The listing builds one solid part. Answer for the finished solid, in the listing's coordinates (mm). Face numbers are marked on the shaded views. A direction names the side the tool comes from. Round coordinates to 2 decimals unless told otherwise and drop trailing zeros. Loops run counter-clockwise (first coordinate to the right, second up) from the corner with the lowest first, then second, coordinate; pieces in that order, holes last. Notation, with made-up numbers: (58, -22) - (84, -22) arc R29 cw to (84, 14) - close; hole circle Ø1 at (-38, 7.25). An arc over 180 degrees is marked (long way). One line per item, written item: value.
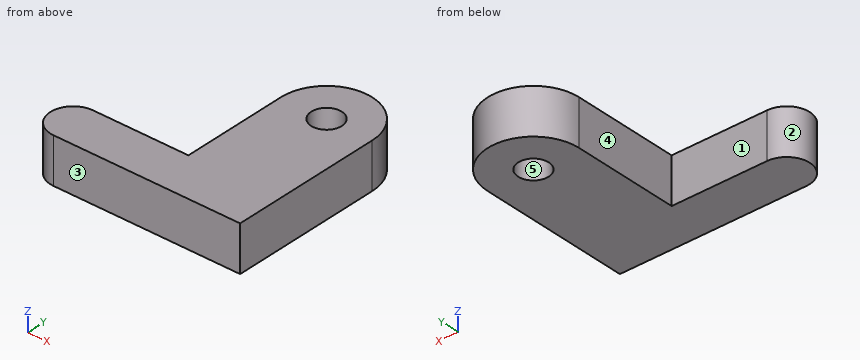
```python
from build123d import *

# Parameters (mm, degrees)
F0_R     = 1
F1_DEPTH = 3


with BuildPart() as f1:
    # F0 (on Top) → F1 (new body)
    with BuildSketch(Plane.XY):
        with BuildLine():
            Line((-6, 3), (-12.259949, 3))
            ThreePointArc((-12.259949, 3), (-13.759949, 1.5), (-12.259949, 0))
            Line((-12.259949, 0), (0, 0))
            Line((0, 0), (0, 10.004636))
            ThreePointArc((0, 10.004636), (-3, 13.004636), (-6, 10.004636))
            Line((-6, 10.004636), (-6, 3))
        make_face()
        with Locations((-3, 10.004636)):
            Circle(F0_R, mode=Mode.SUBTRACT)
    extrude(amount=F1_DEPTH)


solid = f1.part
```
1) A cutting plane is placed at B-B on x = -3. Give the vertices of the cut face in (y, z).
Final values:
outline: (0, 0) - (9, 0) - (9, 3) - (0, 3) - close; (11, 0) - (13, 0) - (13, 3) - (11, 3) - close
2) A cutting plane is placed at D-D on x = -11. Give the vertices of the cut face in (y, z), and give its area (3 significant figures).
Final values:
outline: (0, 0) - (3, 0) - (3, 3) - (0, 3) - close
area: 9.00 mm2
3) Consider L1, parallel to Y at x = -3, z = 0.8; L2, parallel to X at y = 5.25, z = 2.5; L3, parallel to X at y = 10.75, z = 1.2. Determine where each line is inside the solid, lowest interval first.
Final values:
L1: 0 to 9, 11 to 13
L2: -6 to 0
L3: -5.91 to -3.67, -2.33 to -0.09
4) Each of these flat-tipped pins is pushed along its axis until it touches: pin 1 Ø1.5 at (x, z) = (-10, 1) entering from +Y; pin 2 Ø1.5 at (y, z) = (5, 1) entering from -X; pin 3 Ø1.5 at (x, z) = (-6.5, 1.5) entering from -Y. Where does it stop, or does it pass through?
Final values:
pin 1: y = 3
pin 2: x = -6
pin 3: y = 0
5) A cutting plane is placed at A-A on z = 1.55. Give the vertices of the cut face in (x, y), and give its area (3 significant figures).
Final values:
outline: (-12.26, 0) - (0, 0) - (0, 10) arc R3 ccw to (-6, 10) - (-6, 3) - (-12.26, 3) arc R1.5 ccw to start; hole circle Ø2 at (-3, 10)
area: 93.3 mm2
6) For the marked faces 1 and 2, determine the directions among +Z, -Z, +X, -X, +Y, -Y from which every point of the face is accessible in a straight line to the end or side of a thin tool.
Final values:
face 1: +Z, -Z, -X, +Y
face 2: +Z, -Z, -X
7) For a pull along Y with two mould halves and no side action, classify the marked faces 3, 4 and 5 as released by +Y, released by -Y, zero draft, split by the parting line, or undercut.
Final values:
face 3: released by -Y
face 4: zero draft
face 5: undercut
8) A cutting plane is placed at C-C on y = 10.5. Give the vertices of the cut face in (x, z), and give its area (3 significant figures).
Final values:
outline: (-5.96, 0) - (-3.87, 0) - (-3.87, 3) - (-5.96, 3) - close; (-2.13, 0) - (-0.04, 0) - (-0.04, 3) - (-2.13, 3) - close
area: 12.5 mm2
